The drawing under review shows one solid part. Ordinate dimensions are in mm from its lowest x, y, z. Coordinates: 2 decimals unless noted, no trailing zeros. Order: outer loops, then holes, each group sorted by start corner. A loop starts at its lowest first (then second) coordinate and runs counter-clockwise, first axis right, second up. Notation, with made-up numbers: (52.5, 63) - (110.5, 63) arc R21 cw to (110.5, 68) - close; hole circle Ø2 at (16, -23.75). An arc over 180 degrees is marked (long way). Write each question's results on one line, items separated by ' | '. Start each with the question number.
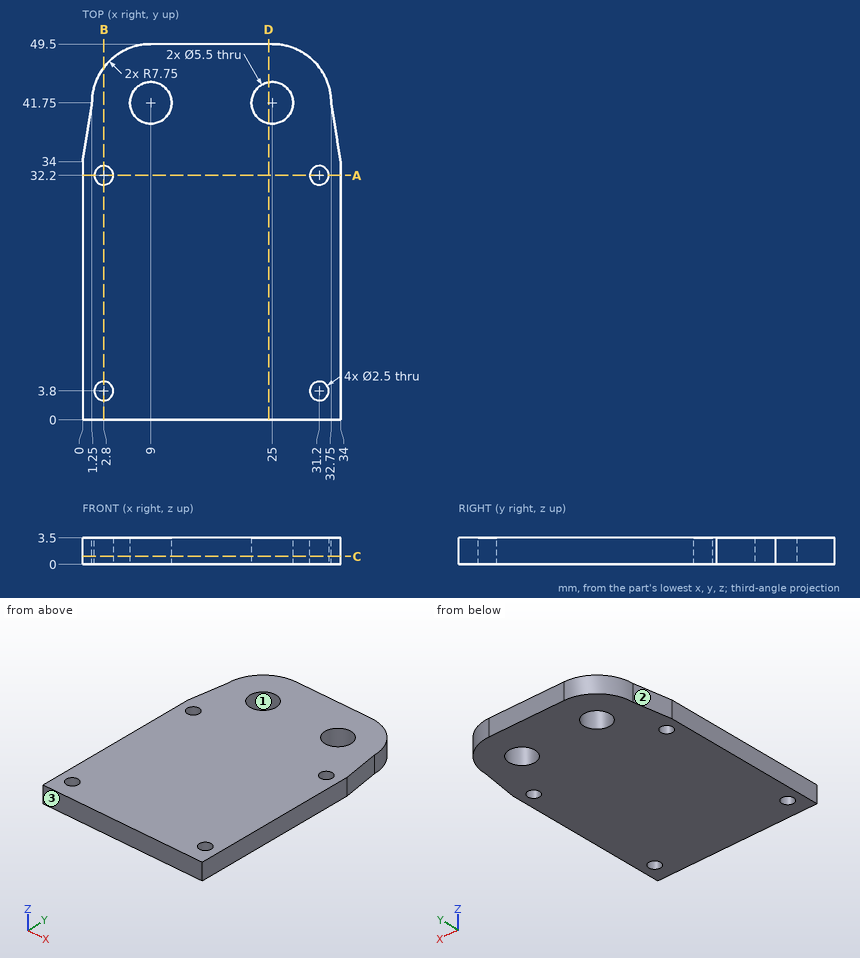
(1) Mouldability with a two-part tool opening along X and no side actions: class the marked faces 1, 2 and 3 as +X half, -X half, draft (parallel to the pull), parting line (faces both ways), or undercut.
(2) Take a section at C-C (z = 1.05). State the section outline as (x, y) points.
(3) Clearance check with flat-ended pins moving along their axes: pin 1 (1.5 mm diameter, centred on x = 2.8, y = 3.8, fed in from -Z) (3 decimals); pin 2 (2 mm diameter, centred on x = 30.5, y = 21.5, fed in from -Z); pin 3 (2 mm diameter, centred on x = 28.5, z = 0.5, fed in from +Y). State where each tip first meets the part, or that it passes through.
(4) Take a section at B-B (x = 2.8). State the section outline as (y, z) points, plus the area to 3 significant figures.
(5) To check wall thickness, follow line 1 along Y through (x, z) = (25, 2.65); line 2 along X through (y, z) = (41.75, 1.75); line 3 along X through (y, z) = (43, 2.15). State the ranges of each line that lie inside material, in increasing order. Write a range as [from, to].
(6) Take a section at D-D (x = 24.5). State the section outline as (y, z) points, plus the area to 3 significant figures.
(7) Take a section at A-A (y = 32.2). State the section outline as (x, z) points.
Worked out:
1) face 1: undercut | face 2: -X half | face 3: draft
2) outline: (0, 0) - (34, 0) - (34, 34) - (32.75, 41.75) arc R7.75 ccw to (25, 49.5) - (9, 49.5) arc R7.75 ccw to (1.25, 41.75) - (0, 34) - close; hole circle Ø2.5 at (2.8, 3.8); hole circle Ø2.5 at (2.8, 32.2); hole circle Ø5.5 at (9, 41.75); hole circle Ø5.5 at (25, 41.75); hole circle Ø2.5 at (31.2, 3.8); hole circle Ø2.5 at (31.2, 32.2)
3) pin 1: through | pin 2: z = 0 | pin 3: y = 49.09
4) outline: (0, 0) - (2.55, 0) - (2.55, 3.5) - (0, 3.5) - close; (5.05, 0) - (30.95, 0) - (30.95, 3.5) - (5.05, 3.5) - close; (33.45, 0) - (46.4, 0) - (46.4, 3.5) - (33.45, 3.5) - close | area: 145 mm^2
5) line 1: [0, 39], [44.5, 49.5] | line 2: [1.25, 6.25], [11.75, 22.25], [27.75, 32.75] | line 3: [1.35, 6.55], [11.45, 22.55], [27.45, 32.65]
6) outline: (0, 0) - (39.05, 0) - (39.05, 3.5) - (0, 3.5) - close; (44.45, 0) - (49.5, 0) - (49.5, 3.5) - (44.45, 3.5) - close | area: 154 mm^2
7) outline: (0, 0) - (1.55, 0) - (1.55, 3.5) - (0, 3.5) - close; (4.05, 0) - (29.95, 0) - (29.95, 3.5) - (4.05, 3.5) - close; (32.45, 0) - (34, 0) - (34, 3.5) - (32.45, 3.5) - close
